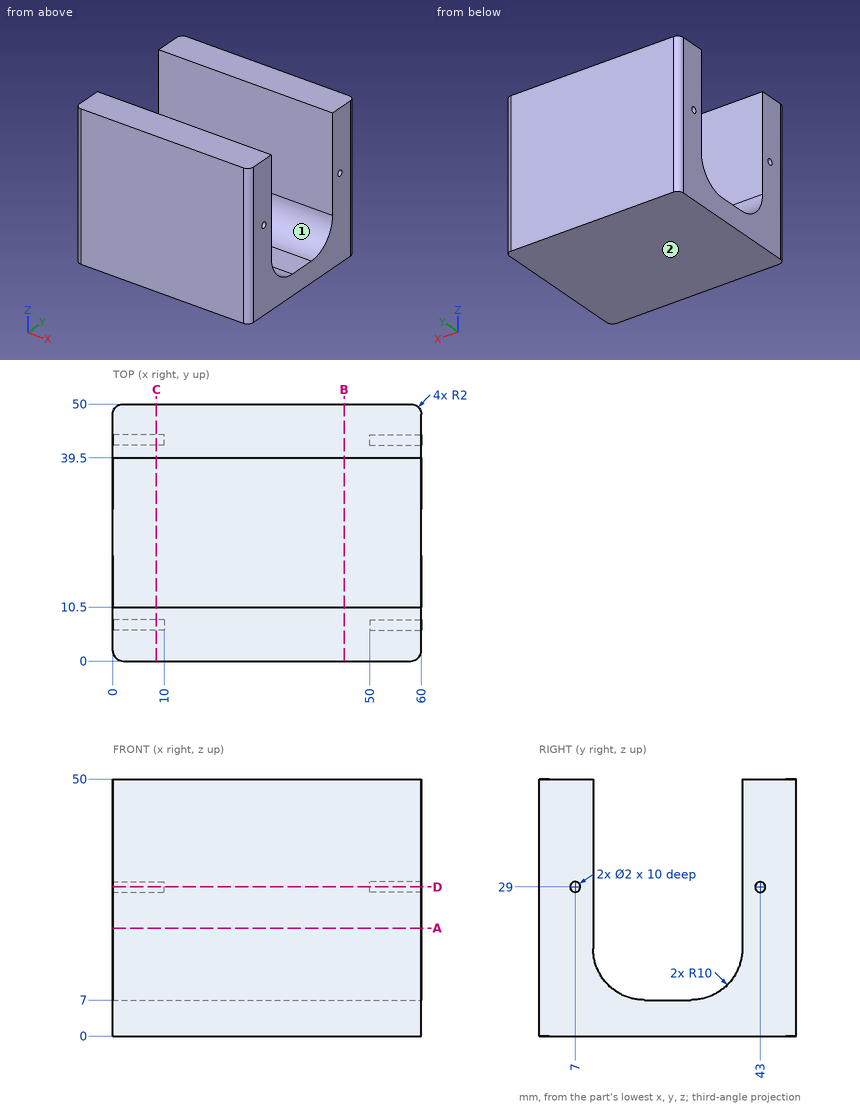
Here's the drawing with two shaded views (mm, measured from the low corner). I have some questions. A direction names the side the tool comes from. Coordinates: 2 decimals unless noted, no trailing zeros. Write each loop counter-clockwise with the first axis right and the second up, starting at its lowest first coordinate (ties: lowest second). Pieces come first, ordered by that corner, then holes. Notation, with made-up numbers: (61.25, 60.25) -> (93.25, 60.25) arc R14 cw to (93.25, 79.25) -> close; hole circle Ø6 at (48.5, 81). An arc over 180 degrees is marked (long way). Use a Markdown table: item, result. Add a question column.
(1) I'm going to push flat-ended pins straight in: P1, Ø8, axis at y = 14, z = 42, coming from the -X side; P2, Ø1.2, axis at y = 43, z = 29, coming from the +X side; P3, Ø0.6, axis at y = 43, z = 28.5, coming from the -X side; P4, Ø4.5, axis at x = 39.5, y = 23.5, coming from the +Z side. Where does each tip first touch, or does it pass through?
(2) For the marked faces 1 and 2, which set-ups out of +Z, -Z, +X, -X, +Y, -Y let a thin tool reach every point of the face, with its end or its side?
(3) Please list where these lines run through material, in increasing order: line 1 (Y direction, x = 7, z = 29); line 2 (Y direction, x = 9, z = 21.5); line 3 (Z direction, x = 56.75, y = 43).
(4) If we section it at A-A, the plane z = 21: Write out the boundary of the cut face in (x, y).
(5) If we section it at D-D, the plane z = 29: Write out the boundary of the cut face in (x, y).
(6) If we section it at C-C, the plane x = 8.5: Write out the boundary of the cut face in (y, z).
(7) If we section it at B-B, the plane x = 45: Write out the boundary of the cut face in (y, z).
Outcome:
| question | item | result |
|---|---|---|
| 1 | P1 | stops at x = 0 |
| 1 | P2 | stops at x = 50 |
| 1 | P3 | stops at x = 10 |
| 1 | P4 | stops at z = 7 |
| 2 | face 1 | +Z, +X, -X |
| 2 | face 2 | -Z, +X, -X, +Y, -Y |
| 3 | line 1 | y = 0 to 6, 8 to 10.5, 39.5 to 42, 44 to 50 |
| 3 | line 2 | y = 0 to 10.5, 39.5 to 50 |
| 3 | line 3 | z = 0 to 28, 30 to 50 |
| 4 | outline | (0, 2) arc R2 ccw to (2, 0) -> (58, 0) arc R2 ccw to (60, 2) -> (60, 10.5) -> (0, 10.5) -> close; (0, 39.5) -> (60, 39.5) -> (60, 48) arc R2 ccw to (58, 50) -> (2, 50) arc R2 ccw to (0, 48) -> close |
| 5 | outline | (0, 2) arc R2 ccw to (2, 0) -> (58, 0) arc R2 ccw to (60, 2) -> (60, 6) -> (50, 6) -> (50, 8) -> (60, 8) -> (60, 10.5) -> (0, 10.5) -> (0, 8) -> (10, 8) -> (10, 6) -> (0, 6) -> close; (0, 39.5) -> (60, 39.5) -> (60, 42) -> (50, 42) -> (50, 44) -> (60, 44) -> (60, 48) arc R2 ccw to (58, 50) -> (2, 50) arc R2 ccw to (0, 48) -> (0, 44) -> (10, 44) -> (10, 42) -> (0, 42) -> close |
| 6 | outline | (0, 0) -> (50, 0) -> (50, 50) -> (39.5, 50) -> (39.5, 17) arc R10 cw to (29.5, 7) -> (20.5, 7) arc R10 cw to (10.5, 17) -> (10.5, 50) -> (0, 50) -> close; hole circle Ø2 at (7, 29); hole circle Ø2 at (43, 29) |
| 7 | outline | (0, 0) -> (50, 0) -> (50, 50) -> (39.5, 50) -> (39.5, 17) arc R10 cw to (29.5, 7) -> (20.5, 7) arc R10 cw to (10.5, 17) -> (10.5, 50) -> (0, 50) -> close |
